Build history of the part. All positions in model axes, mm. A direction names the side the tool comes from. Give positions to 0.01 mm unless a question says otherwise; leave off trailing zeros. Order: outer loops, then holes, each group sorted by start corner. A loop starts at its lowest first (then second) coordinate and runs counter-clockwise, first axis right, second up. Notation, with made-up numbers: (-0.5, 89.5) - (52.5, 89.5) arc R27 ccw to (52.5, 123.5) - close; hole circle Ø10 at (-34.5, 38). An arc over 180 degrees is marked (long way). Use a Markdown table: item, result.
from build123d import *

# Parameters (mm, degrees)
SKETCH1_R           = 2.5
BOSS_EXTRUDE1_DEPTH = 43.02


with BuildPart() as part:
    # Sketch1 → Boss-Extrude1 (new body)
    with BuildSketch(Plane.XY):
        Circle(SKETCH1_R)
    extrude(amount=BOSS_EXTRUDE1_DEPTH)

    # Sketch3 → #6-40 Tapped Hole1 (revolve, cut)
    with BuildSketch(Plane(origin=(0, 0, 43.02), x_dir=(0, -1, 0), z_dir=(1, 0, 0))):
        Polygon((0, 0), (0, 9.782295074), (1.4351, 8.92), (1.4351, 0.799242399), (2.3876, 0), align=None)
    f_6_40_tapped_hole1 = revolve(axis=Axis((0, 0, 49.37), (0, 0, -1)), mode=Mode.SUBTRACT)

    # Mirror1: #6-40 Tapped Hole1 across plane
    add(f_6_40_tapped_hole1.mirror(Plane.XY.offset(21.51)), mode=Mode.SUBTRACT)


solid = part.part
1) Wall check: line 1 (Y direction, x = 0, z = 39.25); line 2 (Y direction, x = -0.5, z = 34.5); line 3 (X direction, y = 0.8, z = 17). Give the ranges that are in metal, low to high. Write a range as from..to.
Computed:
| item | result |
|---|---|
| line 1 | y = -2.5..-1.44, 1.44..2.5 |
| line 2 | y = -2.45..-1.35, 1.35..2.45 |
| line 3 | x = -2.37..2.37 |
2) Two-plate mould, pull along Y, no slides. Class faces 3 (the conical face through (0.243, 0.054, 33.387)), 4 (the cylindrical face through (0.87, 1.14, 4.8)), 5 (the cylindrical face through (-0.54, -2.44, 21.21)): +Y half, -Y half, draft (parallel to the pull), parting line (faces both ways), or undercut.
Computed:
| item | result |
|---|---|
| face 3 | undercut |
| face 4 | undercut |
| face 5 | parting line |
3) Tool access for faces 1 (the cylindrical face through (0.87, 1.14, 38.22)), 2 (the conical face through (0.243, 0.054, 9.633)): list every direction of +Z, -Z, +X, -X, +Y, -Y with a clear straight run to the whole face (end or side of a thin tool).
Computed:
| item | result |
|---|---|
| face 1 | +Z |
| face 2 | -Z |
4) Slice it at A-A (z = 17.5). Write the cut outline in (x, y).
Computed:
| item | result |
|---|---|
| outline | circle Ø5 at (0, 0) |
5) Pin check, flat tips, straight feed: P1, Ø1, axis at x = -0.5, y = -1, coming from the +Z side; P2, Ø1, axis at y = -1.5, z = 8.5, coming from the -X side; P3, Ø2, axis at x = -1, z = 20, coming from the -Y side; P4, Ø1.7, axis at x = 0, y = 0, coming from the -Z side. Stop position of each tip, or through.
Computed:
| item | result |
|---|---|
| P1 | stops at z = 42.37 |
| P2 | stops at x = -2.29 |
| P3 | stops at y = -2.5 |
| P4 | stops at z = 9.27 |
